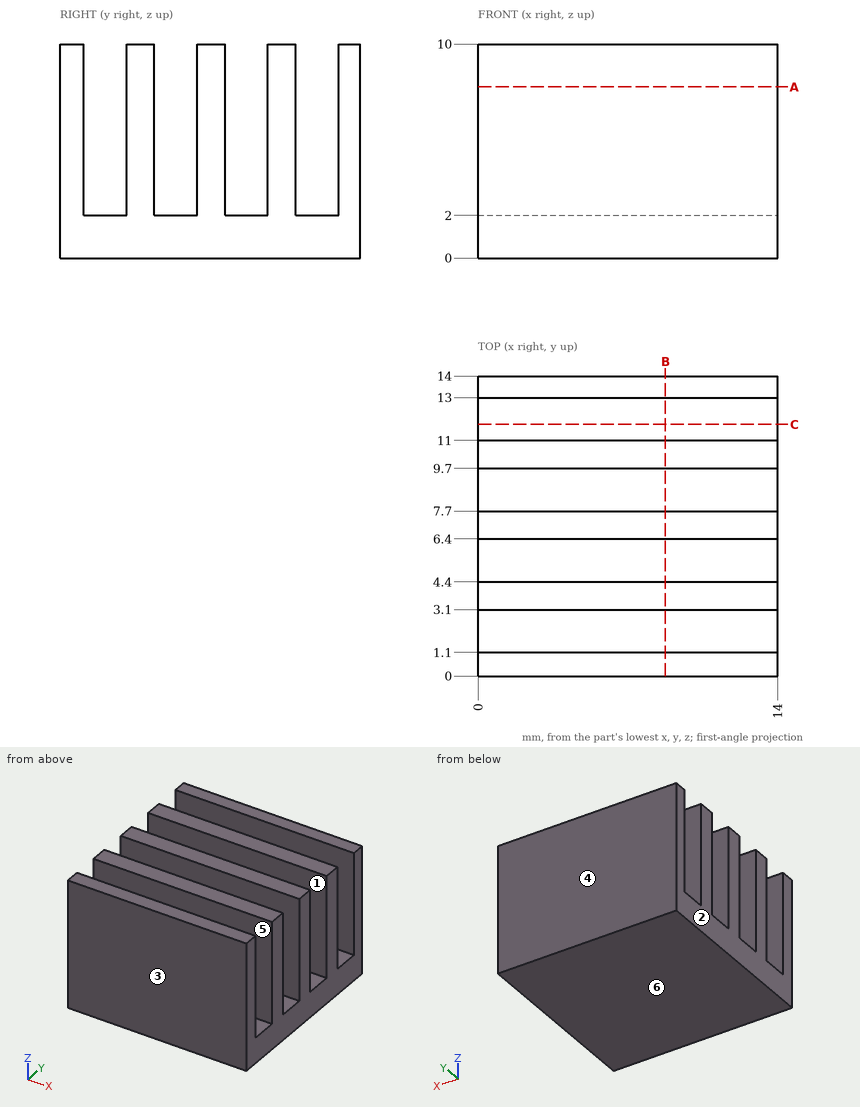
The figure shows three views and two pictorial views of one solid part (mm, origin at its lowest corner). Answer the questions. A direction names the side the tool comes from. Coordinates: 2 decimals unless noted, no trailing zeros. Write each loop counter-clockwise with the first axis right and the second up, starting at its lowest first coordinate (ties: lowest second). Pieces come first, ordered by that corner, then holes.
1. For the marked faces 1 and 2, determine the directions among +Z, -Z, +X, -X, +Y, -Y from which every point of the face is accessible in a straight line to the end or side of a thin tool.
Results list:
face 1: +Z, +X, -X
face 2: +Z, -Z, -X, +Y, -Y
2. For a pull along Y with two mould halves and no side action, classify the marked faces 3, 4, 5 and 6 as +Y half, -Y half, draft (parallel to the pull), parting line (faces both ways), or undercut.
Results list:
face 3: -Y half
face 4: +Y half
face 5: undercut
face 6: draft
3. The part is cut by section A-A, the plane z = 8. Write down the section's boundary in (x, y).
Results list:
outline: (0, 0) - (14, 0) - (14, 1.1) - (0, 1.1) - close; (0, 3.1) - (14, 3.1) - (14, 4.4) - (0, 4.4) - close; (0, 6.4) - (14, 6.4) - (14, 7.7) - (0, 7.7) - close; (0, 9.7) - (14, 9.7) - (14, 11) - (0, 11) - close; (0, 13) - (14, 13) - (14, 14) - (0, 14) - close
4. Consider line 1 along Y through (x, z) = (7.25, 2.25); line 2 along Z through (x, y) = (3, 11.5). Determine where each line is inside the solid, lowest interval first.
Results list:
line 1: y = 0 to 1.1, 3.1 to 4.4, 6.4 to 7.7, 9.7 to 11, 13 to 14
line 2: z = 0 to 2
5. The part is cut by section B-B, the plane x = 8.75. Write down the section's boundary in (y, z).
Results list:
outline: (0, 0) - (14, 0) - (14, 10) - (13, 10) - (13, 2) - (11, 2) - (11, 10) - (9.7, 10) - (9.7, 2) - (7.7, 2) - (7.7, 10) - (6.4, 10) - (6.4, 2) - (4.4, 2) - (4.4, 10) - (3.1, 10) - (3.1, 2) - (1.1, 2) - (1.1, 10) - (0, 10) - close
6. The part is cut by section C-C, the plane y = 11.75. Write down the section's boundary in (x, z), and give its area (3 significant figures).
Results list:
outline: (0, 0) - (14, 0) - (14, 2) - (0, 2) - close
area: 28.0 mm2
7. Flat-ended cylindrical pins translate along their axes: pin 1 (2 mm diameter, centred on x = 4.5, y = 8.5, fed in from +Z); pin 2 (0.6 mm diameter, centred on x = 7, y = 5.5, fed in from +Z). Find the tip coordinate at first contact, or state that the pin passes through.
Results list:
pin 1: stops at z = 10
pin 2: stops at z = 2
